```python
from build123d import *

# Parameters (mm, degrees)
CHAMFER1_SIZE              = 2
CHAMFER2_SIZE              = 2
F_6_0_204_DIAMETER_HOLE1_D = 5.1816
CIRPATTERN1_COUNT          = 6
FILLET2_R                  = 5
FILLET3_R                  = 2


with BuildPart() as part:
    # Sketch2 → Revolve1 (revolve)
    with BuildSketch(Plane(origin=(0, 0, 0), x_dir=(0, 0, -1), z_dir=(1, 0, 0)), mode=Mode.PRIVATE) as revolve1_sk:
        Polygon((-5, 83), (-35, 74.961524227), (-35, 72.961524227), (0, 72.961524227), (0, 49.1), (5, 49.1), (5, 77.5), (25, 77.5), (25, 80), (5, 80), (5, 83), align=None)
    revolve(revolve1_sk.sketch.rotate(Axis((0, 0, -77), (0, 0, 1)), 90), axis=Axis((0, 0, -77), (0, 0, 1)))

    # Chamfer1
    chamfer1_edges = [part.edges().sort_by_distance(p)[0] for p in [
        (77.5, 0, -25),
    ]]
    chamfer(chamfer1_edges, length=CHAMFER1_SIZE)

    # Chamfer2
    chamfer2_edges = [part.edges().sort_by_distance(p)[0] for p in [
        (49.1, 0, 0),
    ]]
    chamfer(chamfer2_edges, length=CHAMFER2_SIZE)

    # #6 (0.204) Diameter Hole1 (through all)
    with Locations(Plane.XY):
        with Locations((-33, 57.15767665)):
            f_6_0_204_diameter_hole1 = Hole(F_6_0_204_DIAMETER_HOLE1_D / 2)

    # CirPattern1: #6 (0.204) Diameter Hole1 ×6 about axis
    cirpattern1_axis = Axis((0, 0, 0), (0, 0, 1))
    for i in range(1, CIRPATTERN1_COUNT):
        add(f_6_0_204_diameter_hole1.rotate(cirpattern1_axis, i * 360 / CIRPATTERN1_COUNT), mode=Mode.SUBTRACT)

    # Fillet2
    fillet2_edges = [part.edges().sort_by_distance(p)[0] for p in [
        (77.5, 0, -5),
    ]]
    fillet(fillet2_edges, radius=FILLET2_R)

    # Fillet3
    fillet3_edges = [part.edges().sort_by_distance(p)[0] for p in [
        (72.961524227, 0, 0),
    ]]
    fillet(fillet3_edges, radius=FILLET3_R)


solid = part.part
```
Part model, mm, in its own coordinate system. A direction names the side the tool comes from. Round coordinates to 2 decimals unless told otherwise and drop trailing zeros. Write each loop counter-clockwise with the first axis right and the second up, starting at its lowest first coordinate (ties: lowest second). Pieces come first, ordered by that corner, then holes. Notation, with made-up numbers: M -33,44 L -22,44 A7 cw -22,55 Z; hole C 28.25,67.25 d5. An arc over 180 degrees is marked long. One line per question, with ' | ' between items.
(1) Two-plate mould, pull along Y, no slides. Class faces 3 (the face through (-43, -68, -5)), 4 (the face through (79.923, -3.517, -14.86)), 5 (the face through (-35.762, 68.756, -16.591)), 6 (the face through (21, -48, 0)): released by +Y, released by -Y, zero draft, split by the parting line, or undercut.
Answer key:
face 3: zero draft | face 4: split by the parting line | face 5: undercut | face 6: undercut
(2) 3-axis set-ups, long thin cutter, end or side, ignore diameter. For faces 1 (the face through (57.9, 44.396, 18.269)), 2 (the face through (-32.44, 54.63, -2.53)): which of +Z, -Z, +X, -X, +Y, -Y reach the whole face in a straight line?
Answer key:
face 1: +Z | face 2: +Z, -Z
(3) Saw through at C-C on z = 17. Write the cut outline in (x, y).
Answer key:
outline: C 0,0 d159.57; hole C 0,0 d145.92
(4) Saw through at B-B on y = 0. Count the separate pieces of the cut face and the enclosed holes in it, then the cut area to 3 significant figures.
Answer key:
separate pieces: 4 | enclosed holes: 0 | area: 853 mm^2
(5) Pin check, flat tips, straight feed: pin 1 (1.5 mm diameter, centred on y = 25.5, z = -16.5, fed in from -X); pin 2 (8.5 mm diameter, centred on x = -33, y = -57.16, fed in from +Z); pin 3 (6.5 mm diameter, centred on x = 66, y = 0, fed in from -Z). Stop position of each tip, or through.
Answer key:
pin 1: stops at x = -76.08 | pin 2: stops at z = 0 | pin 3: stops at z = -5
(6) Probe line 1 along Y through (x, z) = (0, -4); line 2 along X through (y, z) = (0.5, 6.5); line 3 along Z through (x, y) = (36, -60.5). List the from-to ranges inside material, lowest first.
Answer key:
line 1: y = -83 to -49.1, 49.1 to 83 | line 2: x = -82.6 to -72.96, 72.96 to 82.6 | line 3: z = -5 to 0
